Answer from the drawing. Dimensions are ordinates in mm from the lowest x, y and z of the part. A direction names the side the tool comes from. Round coordinates to 2 decimals unless told otherwise and drop trailing zeros. Loops run counter-clockwise (first coordinate to the right, second up) from the corner with the lowest first, then second, coordinate; pieces in that order, holes last. Notation, with made-up numbers: (-38.75, -22.5) - (-17.75, -22.5) arc R27 cw to (-17.75, 1.5) - close; hole circle Ø10 at (-3, 1.25). An arc over 180 degrees is marked (long way). Write item = value, one per line. Start each with the question number.
1) Straight lines are drawn through the part: line 1 along Y through (x, z) = (26.5, 4) (3 decimals); line 2 along Z through (x, y) = (145, 51.5); line 3 along Y through (x, z) = (74, 14) (3 decimals). For each, find the intervals that lie inside material, in ascending order.
2) Section B-B, the plane z = 12 is taken. Determine the outline of the cut face in (x, y) (3 decimals).
3) Section D-D, the plane x = 12 is taken. Determine the outline of the cut face in (y, z) (3 decimals), and give its area (3 significant figures).
4) Section C-C, the plane y = 27 is taken. Determine the outline of the cut face in (x, z).
5) Section A-A, the plane x = 30 is taken. Determine the outline of the cut face in (y, z) (3 decimals).
6) Given pin 1 Ø2.5 at (x, y) = (71, 1) entering from -Z; pin 2 Ø1.2 at (x, z) = (52, 12.5) entering from -Y (3 decimals); pin 3 Ø1.5 at (y, z) = (13, 15.5) entering from -X; pin 4 Ø2 at (y, z) = (30, 8.5) entering from +X, each flat-ended and moving along its own axis, determine where each tip first touches the part or whether it passes through.
7) A tool of negligible diameter and unlimited length cuts with its end or side. For the marked faces 1 and 2, from which of +Z, -Z, +X, -X, +Y, -Y can it reach the whole face along a straight path? Write none if from no direction.
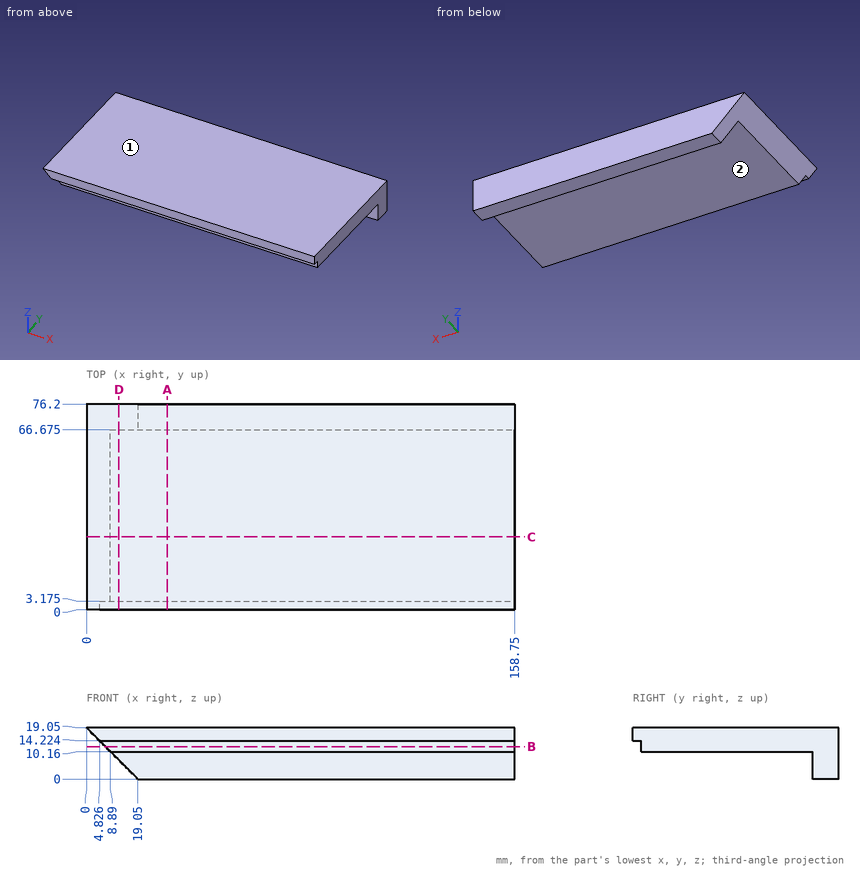
Geometry check:
q1.line_1 = 66.675 to 76.2
q1.line_2 = 10.16 to 19.05
q1.line_3 = 3.175 to 76.2
q2.outline = (7.05, 3.175) - (158.75, 3.175) - (158.75, 76.2) - (7.05, 76.2) - close
q3.outline = (0, 14.224) - (3.175, 14.224) - (3.175, 10.16) - (66.675, 10.16) - (66.675, 7.05) - (76.2, 7.05) - (76.2, 19.05) - (0, 19.05) - close
q3.area = 694 mm2
q4.outline = (0, 19.05) - (8.89, 10.16) - (158.75, 10.16) - (158.75, 19.05) - close
q5.outline = (0, 14.224) - (3.175, 14.224) - (3.175, 10.16) - (66.675, 10.16) - (66.675, 0) - (76.2, 0) - (76.2, 19.05) - (0, 19.05) - close
q6.pin_1 = 14.22
q6.pin_2 = 3.175
q6.pin_3 = 2.8
q6.pin_4 = through
q7.face_1 = +Z, +X, -X, +Y, -Y
q7.face_2 = -Z, +X, -X, -Y
